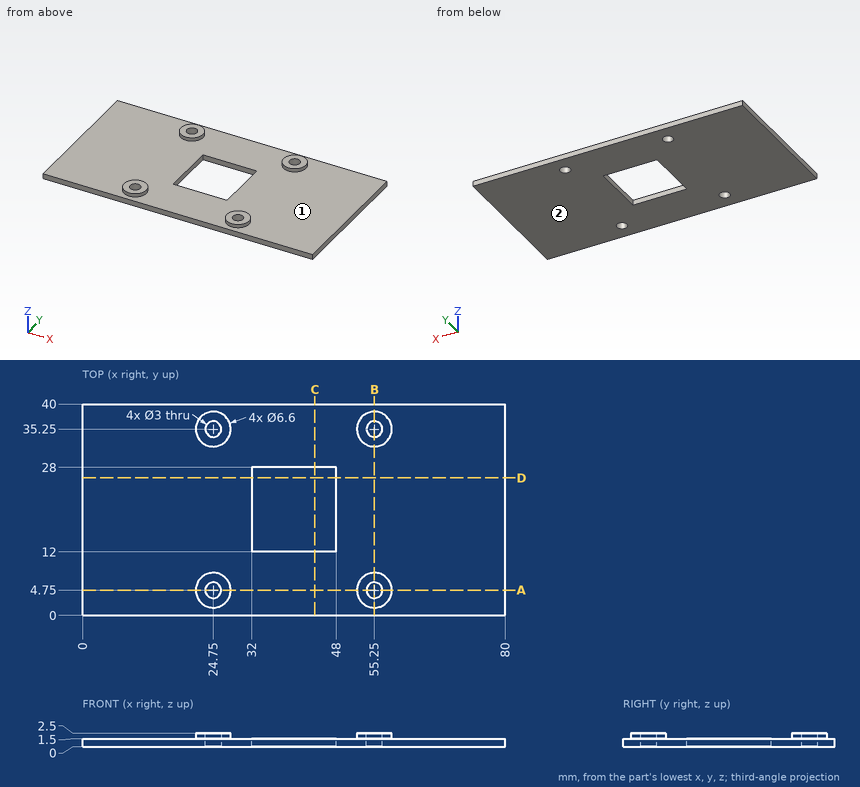
The drawing under review shows one solid part. Ordinate dimensions are in mm from its lowest x, y, z. Round coordinates to 2 decimals unless told otherwise and drop trailing zeros. Write each loop counter-clockwise with the first axis right and the second up, starting at its lowest first coordinate (ties: lowest second). Pieces come first, ordered by that corner, then holes. Notation, with made-up numbers: M 34.25,16 L 64.25,16 A19 ccw 64.25,27 Z; hole C 6,-40 d9. An arc over 180 degrees is marked long. One line per item, written item: value. Start each with the question number.
(1) We need section D-D (y = 26). Give the boundary of the cut face in (x, z), and give its area (3 significant figures).
(2) The part is to be moulded in two halves that separate along Y. For the marked faces 1 and 2, say which applies: released by +Y, released by -Y, zero draft, split by the parting line, or undercut.
(3) Wall thickness on line 1 (Y direction, x = 24.75, z = 1.65); line 2 (X direction, y = 27, z = 1.45); line 3 (Y direction, x = 46.5, z = 1): over which ranges is each line inside the solid? List them lowest first.
(4) We need section B-B (x = 55.25). Give the boundary of the cut face in (y, z), and give its area (3 significant figures).
(5) We need section C-C (x = 44). Give the boundary of the cut face in (y, z).
(6) Insertion check: pin 1 (4 mm diameter, centred on x = 14.5, y = 15, fed in from +Z). The pin has a flat end and moves straight along its axis. Give the tip position at first contact, or say it passes through.
(7) We need section A-A (y = 4.75). Give the boundary of the cut face in (x, z).
Result:
1. outline: M 0,0 L 32,0 L 32,1.5 L 0,1.5 Z; M 48,0 L 80,0 L 80,1.5 L 48,1.5 Z
1. area: 96.0 mm²
2. face 1: undercut
2. face 2: zero draft
3. line 1: 1.45 to 3.25, 6.25 to 8.05, 31.95 to 33.75, 36.75 to 38.55
3. line 2: 0 to 32, 48 to 80
3. line 3: 0 to 12, 28 to 40
4. outline: M 0,0 L 3.25,0 L 3.25,2.5 L 1.45,2.5 L 1.45,1.5 L 0,1.5 Z; M 6.25,0 L 33.75,0 L 33.75,2.5 L 31.95,2.5 L 31.95,1.5 L 8.05,1.5 L 8.05,2.5 L 6.25,2.5 Z; M 36.75,0 L 40,0 L 40,1.5 L 38.55,1.5 L 38.55,2.5 L 36.75,2.5 Z
4. area: 58.2 mm²
5. outline: M 0,0 L 12,0 L 12,1.5 L 0,1.5 Z; M 28,0 L 40,0 L 40,1.5 L 28,1.5 Z
6. pin 1: z = 1.5
7. outline: M 0,0 L 23.25,0 L 23.25,2.5 L 21.45,2.5 L 21.45,1.5 L 0,1.5 Z; M 26.25,0 L 53.75,0 L 53.75,2.5 L 51.95,2.5 L 51.95,1.5 L 28.05,1.5 L 28.05,2.5 L 26.25,2.5 Z; M 56.75,0 L 80,0 L 80,1.5 L 58.55,1.5 L 58.55,2.5 L 56.75,2.5 Z
